Model file for the job. Use its own axes, mm. Give positions to 0.01 mm unless a question says otherwise; leave off trailing zeros. Order: outer loops, then holes, each group sorted by start corner. A loop starts at its lowest first (then second) coordinate and runs counter-clockwise, first axis right, second up. Notation, with made-up numbers: (-36, 72) - (15, 72) arc R25 ccw to (15, 90) - close; hole circle Ø4 at (-1.5, -9.75). An arc over 180 degrees is marked (long way). Return JSON: item names as keys, results as strings. Group by question number.
from build123d import *

# Parameters (mm, degrees)
F0_R     = 75
F1_DEPTH = 10
F3_D     = 13.2


with BuildPart() as f1:
    # F0 (on Front) → F1 (new body)
    with BuildSketch(Plane.XZ):
        Circle(F0_R)
        with BuildLine():
            ThreePointArc((0, 40), (28.2842712475, 28.2842712475), (40, 0))
            ThreePointArc((40, 0), (-28.2842712475, -28.2842712475), (0, 40))
        make_face(mode=Mode.SUBTRACT)
    extrude(amount=F1_DEPTH)

    # F3 (through all)
    with Locations(Plane.XZ.offset(10)):
        with Locations((-44, 44), (-44, -44), (44, -44), (44, 44)):
            Hole(F3_D / 2)


solid = f1.part
(1) Slice it at A-A (z = 44). Give the cut face in (x, y).
(2) Pull direction X, two halves, no side cores. Call faces 1 (the face through (37.903, -4.93, 41.472)), 2 (the face through (-9.764, -4.93, 74.362)), 3 (the face through (32, 0, -32)): released by +X, released by -X, zero draft, split by the parting line, or undercut.
(3) Slice it at D-D (z = -27). Give the cut face in (x, y), and give its area (3 significant figures).
(4) Slice it at B-B (x = -21). Give the cut face in (y, z).
(5) Slice it at C-C (y = -3.25). Give the cut face in (x, z).
(6) Drill centre lines: L1, parallel to Z at x = -44, y = -5.5; L2, parallel to X at y = -7.75, z = 47. Where is each one in solid material? Low to high.
(7) Drop flat-ended pins along their axis: pin 1 Ø1.5 at (x, y) = (31, -8) entering from -Z; pin 2 Ø1 at (y, z) = (-6, 55.5) entering from -X; pin 3 Ø8 at (x, z) = (28.5, 38.5) entering from +Y; pin 4 Ø5 at (x, y) = (57.5, -5) entering from -Z. Give the stop position or say it passes through.
Result set:
{
 "1": {"outline": "(-60.74, -10) - (-50.6, -10) - (-50.6, 0) - (-60.74, 0) - close; (-37.4, -10) - (37.4, -10) - (37.4, 0) - (-37.4, 0) - close; (50.6, -10) - (60.74, -10) - (60.74, 0) - (50.6, 0) - close"},
 "2": {"face 1": "undercut", "face 2": "split by the parting line", "face 3": "zero draft"},
 "3": {"outline": "(-69.97, -10) - (-29.51, -10) - (-29.51, 0) - (-69.97, 0) - close; (29.51, -10) - (69.97, -10) - (69.97, 0) - (29.51, 0) - close", "area": "809 mm²"},
 "4": {"outline": "(-10, -72) - (0, -72) - (0, -34.04) - (-10, -34.04) - close; (-10, 34.04) - (0, 34.04) - (0, 72) - (-10, 72) - close"},
 "5": {"outline": "circle Ø150 at (0, 0); hole circle Ø13.2 at (-44, -44); hole circle Ø13.2 at (-44, 44); hole circle Ø80 at (0, 0); hole circle Ø13.2 at (44, -44); hole circle Ø13.2 at (44, 44)"},
 "6": {"L1": "z = -60.74 to -50.6, -37.4 to 37.4, 50.6 to 60.74", "L2": "x = -58.45 to -49.88, -38.12 to 38.12, 49.88 to 58.45"},
 "7": {"pin 1": "stops at z = -68.63", "pin 2": "stops at x = -50.99", "pin 3": "stops at y = 0", "pin 4": "stops at z = -50.99"}
}
